Here's how the part is built. I have some questions about the finished solid (model axes, mm). A direction names the side the tool comes from. Coordinates: 2 decimals unless noted, no trailing zeros. Loops run counter-clockwise (first coordinate to the right, second up) from the corner with the lowest first, then second, coordinate; pieces in that order, holes last. Notation, with made-up numbers: M 37,-2 L 76,-2 A20 cw 76,15 Z; hole C 58.25,67 d5. An arc over 180 degrees is marked long. Use CSV: the item, a comma, the result in double quotes. Start each with the question number.
Q1. If we mould it in two halves opening along X, with no side actions, what happens to faces 1 (the cylindrical face through (27.893, -21.437, 2.465)), 2 (the flat face through (21.88, -3.24, 2.46)), 3 (the flat face through (0, -13.39, -17)), 4 (the flat face through (-24, -13, 0))? For each: +X half, -X half, draft (parallel to the pull), parting line (faces both ways), or undercut.
Q2. If we section it at D-D (x = -14): Please give me the cut outline in (y, z).
Q3. For pin 1 Ø8 at (x, z) = (-5.5, -7.5) entering from +Y; pin 2 Ø1.3 at (y, z) = (-12, -14) entering from -X; pin 3 Ø0.8 at (y, z) = (-12.5, -27.5) entering from +X; pin 4 Ø13 at (x, y) = (0, 36.79) entering from +Z, each with a flat end and sliding along its axis, tell me the tip position at first contact or that it passes through.
Q4. Please list where these lines run through material, in increasing order: probe 1 along Z at (x, y) = (21.5, -15.5); probe 2 along Y at (x, z) = (4, -12); probe 3 along X at (y, z) = (-12.5, -37.5). Write a range as [from, to].
Q5. If we section it at A-A (x = 0): Please give me the cut outline in (y, z) (3 decimals), and give its area (3 significant figures).
Q6. Which directions (+Z, -Z, +X, -X, +Y, -Y) give clear straight access to the entire face, cutting with the end or side of a thin tool? Please do faces 5 (the flat face through (-2.27, -12, -17)), 6 (the flat face through (-8.21, 25, 2)), 7 (the flat face through (8.21, 25, 2)), 8 (the cylindrical face through (0, 45, 2)).
Q7. If we section it at B-B (y = -4.5): Please give me the cut outline in (x, z).
Q8. If we section it at C-C (z = -21): Please give me the cut outline in (x, y) (3 decimals).
from build123d import *
from build123d.topology import SkipClean

# Parameters (mm, degrees)
SZKIC1_R                    = 5
SZKIC1_R_2                  = 11.115
DODANIE_WYCI_GNI_CIE1_DEPTH = 5
DODANIE_WYCI_GNI_CIE2_START = 40
SZKIC2_R                    = 16.115
SZKIC2_R_2                  = 11.115
DODANIE_WYCI_GNI_CIE2_DEPTH = 40
WYTNIJ_WYCI_GNI_CIE1_DEPTH  = 76.204328466
WYTNIJ_WYCI_GNI_CIE2_DEPTH  = 73.323516369


with BuildPart() as part:
    # Szkic1 → Dodanie-wyciągnięcie1 (new body)
    with BuildSketch(Plane.XY):
        with BuildLine():
            Line((35.966074605, -11.284931435), (27.812788277, -6.577629379))
            ThreePointArc((27.812788277, -6.577629379), (24.75100604, 14.29), (8.21, 27.375395888))
            Line((8.21, 27.375395888), (8.21, 36.79))
            ThreePointArc((8.21, 36.79), (0, 45), (-8.21, 36.79))
            Line((-8.21, 36.79), (-8.21, 27.375395888))
            ThreePointArc((-8.21, 27.375395888), (-24.75100604, 14.29), (-27.812788277, -6.577629379))
            Line((-27.812788277, -6.577629379), (-35.966074605, -11.284931435))
            ThreePointArc((-35.966074605, -11.284931435), (-38.97114317, -22.5), (-27.756074605, -25.505068565))
            Line((-27.756074605, -25.505068565), (-19.602788277, -20.797766509))
            ThreePointArc((-19.602788277, -20.797766509), (0, -28.58), (19.602788277, -20.797766509))
            Line((19.602788277, -20.797766509), (27.756074605, -25.505068565))
            ThreePointArc((27.756074605, -25.505068565), (38.97114317, -22.5), (35.966074605, -11.284931435))
        make_face()
        with Locations((0, 36.79)):
            Circle(SZKIC1_R, mode=Mode.SUBTRACT)
        with Locations((31.861074605, -18.395)):
            Circle(SZKIC1_R, mode=Mode.SUBTRACT)
        with Locations((-31.861074605, -18.395)):
            Circle(SZKIC1_R, mode=Mode.SUBTRACT)
        Circle(SZKIC1_R_2, mode=Mode.SUBTRACT)
    extrude(amount=DODANIE_WYCI_GNI_CIE1_DEPTH)

    # Szkic2 → Dodanie-wyciągnięcie2 (add)
    with SkipClean():  # the faces are left unmerged after this step: merging them gives an invalid solid
        with BuildSketch(Plane(origin=(0, 0, 0), x_dir=(-1, 0, 0), z_dir=(0, 0, -1)).offset(DODANIE_WYCI_GNI_CIE2_START)):
            with Locations(Location((0, 0, 0), (0, 0, 180))):
                Circle(SZKIC2_R)
            Circle(SZKIC2_R_2, mode=Mode.SUBTRACT)
        extrude(amount=-DODANIE_WYCI_GNI_CIE2_DEPTH)

    # Szkic3 → Wytnij-wyciągnięcie1 (cut, through all)
    with BuildSketch(Plane.XY.offset(5)):
        Polygon((2.27, -10.880731823), (2.27, -7.598635721), (-2.27, -7.598635721), (-2.27, -10.880731823), (-2.27, -13.39), (2.27, -13.39), align=None)
    extrude(amount=-WYTNIJ_WYCI_GNI_CIE1_DEPTH, mode=Mode.SUBTRACT)

    # Szkic4 → Wytnij-wyciągnięcie2 (cut, through all)
    with SkipClean():  # the faces are left unmerged after this step: merging them gives an invalid solid
        with BuildSketch(Plane(origin=(0, 0, 0), x_dir=(-1, 0, 0), z_dir=(0, 0, -1))):
            with BuildLine():
                Line((19.602788277, -20.797766509), (7.904031757, -14.043486283))
                ThreePointArc((7.904031757, -14.043486283), (0, -16.115), (-7.904031757, -14.043486283))
                Line((-7.904031757, -14.043486283), (-19.602788277, -20.797766509))
                ThreePointArc((-19.602788277, -20.797766509), (0, -28.58), (19.602788277, -20.797766509))
            make_face()
            with BuildLine():
                Line((27.812788277, -6.577629379), (16.115, 0))
                ThreePointArc((16.115, 0), (13.999953125, 7.980885759), (8.21, 13.866835436))
                Line((8.21, 13.866835436), (8.21, 27.375395888))
                ThreePointArc((8.21, 27.375395888), (24.75100604, 14.29), (27.812788277, -6.577629379))
            make_face()
            with BuildLine():
                Line((-8.21, 27.375395888), (-8.21, 13.866835436))
                ThreePointArc((-8.21, 13.866835436), (-13.999953125, 7.980885759), (-16.115, 0))
                Line((-16.115, 0), (-27.812788277, -6.577629379))
                ThreePointArc((-27.812788277, -6.577629379), (-24.75100604, 14.29), (-8.21, 27.375395888))
            make_face()
        extrude(amount=-WYTNIJ_WYCI_GNI_CIE2_DEPTH, mode=Mode.SUBTRACT)


solid = part.part
Results below:
1,face 1,"undercut"
1,face 2,"+X half"
1,face 3,"undercut"
1,face 4,"draft"
2,outline,"M -17.56,0 L -7.98,0 L -7.98,-40 L 7.98,-40 L 7.98,5 L -17.56,5 Z"
3,pin 1,"y = 16.05"
3,pin 2,"x = -11.44"
3,pin 3,"x = 10.64"
3,pin 4,"z = 5"
4,probe 1,"[0, 5]"
4,probe 2,"[-15.61, -10.37], [10.37, 15.61]"
4,probe 3,"[-10.17, -2.27], [2.27, 10.17]"
5,outline,"M -16.115,-40 L -13.39,-40 L -13.39,5 L -16.115,5 Z; M 11.115,-40 L 16.115,-40 L 16.115,0 L 31.79,0 L 31.79,5 L 11.115,5 Z; M 41.79,0 L 45,0 L 45,5 L 41.79,5 Z"
5,area,"442 mm^2"
6,face 5,"+Z, -Z"
6,face 6,"+Z, -Z, -X, +Y"
6,face 7,"+Z, -Z, +X, +Y"
6,face 8,"+Z, -Z, +Y"
7,outline,"M -24.12,0 L -15.47,0 L -15.47,-40 L -10.16,-40 L -10.16,5 L -24.12,5 Z; M 10.16,-40 L 15.47,-40 L 15.47,0 L 24.12,0 L 24.12,5 L 10.16,5 Z"
8,outline,"C 0,0 d32.23; hole M -2.27,-13.39 L 2.27,-13.39 L 2.27,-10.881 A11.115 ccw long -2.27,-10.881 Z"
